Geometry: final body of the model. Coordinates: model frame, mm. Give positions to 0.01 mm unless a question says otherwise; leave off trailing zeros. Write each loop counter-clockwise with the first axis right and the second up, starting at its lowest first coordinate (ties: lowest second). Pieces come first, ordered by that corner, then holes. Notation, with made-up numbers: (61, -18) -> (79, -18) arc R21 cw to (79, 15) -> close; hole circle Ø4 at (25, 70). An arc over 180 degrees is marked (long way). Answer in a Markdown table with one row per item. Add a question column.
Item 1: Draft query along X for faces 1 (the flat face through (0, 64, 7.785)), 2 (the flat face through (1, 1, 0)), 3 (the conical face through (-11.843, -53.334, 0.59)), 4 (the flat face through (1, 1, 2.54)). Return one class per face: +X half, -X half, draft (parallel to the pull), parting line (faces both ways), or undercut.
Item 2: Section query A-A on y = 0. Output: boundary loops of the cut face in (x, z).
Item 3: First-contact query: P1, Ø4, axis at y = 45, z = 7.5, coming from the -X side; P2, Ø7, axis at x = 3, y = -64, coming from the -Z side; P3, Ø5, axis at x = -2.5, y = 58.5, coming from the +Z side. Flat tips, straight axial feed; report the tip coordinate or a pass-through.
Item 4: Section query B-B on x = 0. Output: boundary loops of the cut face in (y, z), plus the area to 3 significant figures.
Item 5: Material intervals for probe 1 along Y at (x, z) = (-14, 7.75); probe 2 along Z at (x, y) = (-26, 39); probe 3 along Y at (x, z) = (-6.5, 8.75), sorted ascending. Write a range as from..to.
```python
from build123d import *

# Parameters (mm, degrees)
F2_T     = -2.54
F3_W     = 22.871588
F3_H     = 2.704573
F4_DEPTH = 69.939388
F5_DEPTH = 69.939388


with BuildPart() as f1:
    # F0 (on Front) → F1 (revolve)
    with BuildSketch(Plane.XZ):
        Polygon((0, 9.426419), (0, 0), (53.611351, 0), (69.938388, 9.426419), align=None)
    revolve(axis=Axis((0, 0, 4.71321), (0, 0, 1)))

    # F2
    f2_openings = [f1.faces().sort_by_distance(p)[0] for p in [
        (0, 0, 9.426419),
    ]]
    offset(amount=F2_T, openings=f2_openings)

    # F3 (on Front) → F4 (cut, through all)
    with BuildSketch(Plane.XZ):
        with Locations((0, 6.432339)):
            Rectangle(F3_W, F3_H)
    extrude(amount=-F4_DEPTH, mode=Mode.SUBTRACT)

    # F3 (on Front) → F5 (cut, through all)
    with BuildSketch(Plane.XZ):
        with Locations((0, 6.432339)):
            Rectangle(F3_W, F3_H)
    extrude(amount=F5_DEPTH, mode=Mode.SUBTRACT)


solid = f1.part
```
Findings below:
| question | item | result |
|---|---|---|
| 1 | face 1 | undercut |
| 1 | face 2 | draft |
| 1 | face 3 | parting line |
| 1 | face 4 | undercut |
| 2 | outline | (-69.94, 9.43) -> (-53.61, 0) -> (53.61, 0) -> (69.94, 9.43) -> (64.86, 9.43) -> (52.93, 2.54) -> (-52.93, 2.54) -> (-64.86, 9.43) -> close |
| 3 | P1 | stops at x = -54 |
| 3 | P2 | stops at z = 4.02 |
| 3 | P3 | stops at z = 5.08 |
| 4 | outline | (-69.94, 9.43) -> (-67.09, 7.78) -> (-62.01, 7.78) -> (-64.86, 9.43) -> close; (-62.41, 5.08) -> (-53.61, 0) -> (53.61, 0) -> (62.41, 5.08) -> (57.33, 5.08) -> (52.93, 2.54) -> (-52.93, 2.54) -> (-57.33, 5.08) -> close; (62.01, 7.78) -> (67.09, 7.78) -> (69.94, 9.43) -> (64.86, 9.43) -> close |
| 4 | area | 326 mm^2 |
| 5 | probe 1 | y = -65.56..-60.35, 60.35..65.56 |
| 5 | probe 2 | z = 0..2.54 |
| 5 | probe 3 | y = -68.46..-63.35, 63.35..68.46 |
